```python
from build123d import *

# Parameters (mm, degrees)
SKETCH1_R            = 62.5
BOSS_EXTRUDE8_DEPTH  = 35
BOSS_EXTRUDE9_REACH  = 192.245
SKETCH2_W            = 15
SKETCH2_H            = 35
FILLET4_R            = 10
FILLET5_R            = 10
SKETCH10_W           = 35
SKETCH10_H           = 15
BOSS_EXTRUDE12_DEPTH = 40
SKETCH6_W            = 35
SKETCH6_H            = 15
BOSS_EXTRUDE10_DEPTH = 40
SKETCH12_W           = 42.229373335
SKETCH12_H           = 20
SKETCH12_W_2         = 40
SKETCH12_H_2         = 15
SKETCH12_W_3         = 39.995847529
BOSS_EXTRUDE13_DEPTH = 97.5
SKETCH13_W           = 20
SKETCH13_H           = 5
SKETCH13_W_2         = 25.5
SKETCH13_H_2         = 5.5
BOSS_EXTRUDE14_DEPTH = 20


with BuildPart() as part:
    # Sketch1 → Boss-Extrude8 (new body)
    with BuildSketch(Plane.XY):
        with BuildLine():
            Line((127.600917431, -117.745016448), (72.5, 0))
            ThreePointArc((72.5, 0), (0, 72.5), (-72.5, 0))
            Line((-72.5, 0), (-127.600917431, -117.745016448))
            Line((-127.600917431, -117.745016448), (-167.600917431, -117.745016448))
            Line((-167.600917431, -117.745016448), (-167.600917431, -137.745016448))
            Line((-167.600917431, -137.745016448), (167.600917431, -137.745016448))
            Line((167.600917431, -137.745016448), (167.600917431, -117.745016448))
            Line((167.600917431, -117.745016448), (127.600917431, -117.745016448))
        make_face()
        with BuildLine():
            ThreePointArc((-67.21559633, -27.171926873), (0, -72.5), (67.21559633, -27.171926873))
            Line((67.21559633, -27.171926873), (101.417450928, -100.25778678))
            Line((101.417450928, -100.25778678), (88.408256881, -117.745016448))
            Line((88.408256881, -117.745016448), (-88.408256881, -117.745016448))
            Line((-88.408256881, -117.745016448), (-101.417450928, -100.25778678))
            Line((-101.417450928, -100.25778678), (-67.21559633, -27.171926873))
        make_face(mode=Mode.SUBTRACT)
        Circle(SKETCH1_R, mode=Mode.SUBTRACT)
    extrude(amount=BOSS_EXTRUDE8_DEPTH)

    # Sketch2 → Boss-Extrude9 (add, up to next)
    with BuildSketch(Plane(origin=(0, -117.745016448, 0), x_dir=(1, 0, 0), z_dir=(0, 1, 0)), mode=Mode.PRIVATE) as boss_extrude9_sk1:
        with Locations((0.093911399, -17.5)):
            Rectangle(SKETCH2_W, SKETCH2_H)
    boss_extrude9_tool1 = extrude(boss_extrude9_sk1.sketch, amount=BOSS_EXTRUDE9_REACH, mode=Mode.PRIVATE) - part.part
    add(boss_extrude9_tool1.solids().sort_by_distance((0.093911, -117.745016, 17.5))[0])

    # Fillet4
    fillet4_edges = [part.edges().sort_by_distance(p)[0] for p in [
        (-167.600917431, -117.745016448, 17.5),
    ]]
    fillet(fillet4_edges, radius=FILLET4_R)

    # Fillet5
    fillet5_edges = [part.edges().sort_by_distance(p)[0] for p in [
        (-127.600917431, -117.745016448, 17.5),
    ]]
    fillet(fillet5_edges, radius=FILLET5_R)

    # Sketch10 → Boss-Extrude12 (add)
    with BuildSketch(Plane(origin=(-72.5, 0, 0), x_dir=(0, 0, -1), z_dir=(1, 0, 0))):
        with Locations((-17.5, -7.5)):
            Rectangle(SKETCH10_W, SKETCH10_H)
    extrude(amount=-BOSS_EXTRUDE12_DEPTH)

    # Sketch6 → Boss-Extrude10 (add)
    with BuildSketch(Plane(origin=(72.5, 0, 0), x_dir=(0, 0, -1), z_dir=(1, 0, 0))):
        with Locations((-17.5, -7.5)):
            Rectangle(SKETCH6_W, SKETCH6_H)
    extrude(amount=BOSS_EXTRUDE10_DEPTH)

    # Sketch12 → Boss-Extrude13 (add)
    with BuildSketch(Plane(origin=(0, 0, 0), x_dir=(-1, 0, 0), z_dir=(0, 0, -1))):
        with Locations((-146.486230764, -127.745016448)):
            Rectangle(SKETCH12_W, SKETCH12_H)
        with Locations((147.600917431, -127.745016448)):
            Rectangle(SKETCH12_W_2, SKETCH12_H)
        with Locations((-92.5, -7.5)):
            Rectangle(SKETCH12_W_2, SKETCH12_H_2)
        with Locations((92.502076235, -7.5)):
            Rectangle(SKETCH12_W_3, SKETCH12_H_2)
    extrude(amount=BOSS_EXTRUDE13_DEPTH)

    # Sketch13 → Boss-Extrude14 (add)
    with BuildSketch(Plane(origin=(0, 0, -97.5), x_dir=(-1, 0, 0), z_dir=(0, 0, -1))):
        with Locations((-92.5, -2.5)):
            Rectangle(SKETCH13_W, SKETCH13_H)
        with Locations((-92.5, -12.5)):
            Rectangle(SKETCH13_W, SKETCH13_H)
        with Locations((92.5, -2.5)):
            Rectangle(SKETCH13_W, SKETCH13_H)
        with Locations((92.5, -12.5)):
            Rectangle(SKETCH13_W, SKETCH13_H)
        with Locations((147.600917431, -120.495016448)):
            Rectangle(SKETCH13_W_2, SKETCH13_H_2)
        with Locations((147.600917431, -134.995016448)):
            Rectangle(SKETCH13_W_2, SKETCH13_H_2)
        with Locations((-147.600917431, -120.495016448)):
            Rectangle(SKETCH13_W_2, SKETCH13_H_2)
        with Locations((-147.600917431, -134.995016448)):
            Rectangle(SKETCH13_W_2, SKETCH13_H_2)
    extrude(amount=BOSS_EXTRUDE14_DEPTH)


solid = part.part
```
CAD build for the part. Positions are in the model's coordinates, mm. A direction names the side the tool comes from. Round coordinates to 2 decimals unless told otherwise and drop trailing zeros. Write each loop counter-clockwise with the first axis right and the second up, starting at its lowest first coordinate (ties: lowest second). Pieces come first, ordered by that corner, then holes. Notation, with made-up numbers: (49, 17) - (97, 17) arc R18 ccw to (97, 42) - close; hole circle Ø7 at (-34.75, -39.5). An arc over 180 degrees is marked (long way). Return JSON: item names as keys, results as strings. Group by question number.
Item 1: Mould opens along Y. For faces 5 (the face through (-1, -72, 35)), 6 (the face through (-128.662, -116.225, 17.745)), 7 (the face through (-92, -7, -97.5)) say: +Y half, -Y half, draft (parallel to the pull), parting line (faces both ways), or undercut.
Item 2: Probe probe 1 along Y at (x, z) = (0, 9); probe 2 along Y at (x, z) = (-55, 5.5); probe 3 along X at (y, z) = (-120, -28). List the from-to ranges inside material, lowest first.
Item 3: Band-saw the part on C-C on z = 14.5. List the corners of the cut face in (x, y).
Item 4: Band-saw the part on B-B on z = -7. List the corners of the cut face in (x, y), plus the area to 3 significant figures.
Item 5: 3-axis set-ups, long thin cutter, end or side, ignore diameter. For faces 1 (the face through (-165, -120, 0)), 2 (the face through (148, -123.245, -107)), 3 (the face through (7.594, -95, 18)), 4 (the face through (93, -15, -40)): which of +Z, -Z, +X, -X, +Y, -Y reach the whole face in a straight line?
Item 6: Band-saw the part on A-A on x = 0. List the corners of the cut face in (y, z), plus the area to 3 significant figures.
Item 7: Band-saw the part on D-D on x = -141. List the corners of the cut face in (y, z), plus the area to 3 significant figures.
Item 8: Flat gauge pins, fed straight in: pin 1 Ø16.5 at (y, z) = (-8.5, -59) entering from -X; pin 2 Ø20 at (x, z) = (-140, -34) entering from +Y (3 decimals); pin 3 Ø6 at (x, z) = (-94, -106) entering from +Y. Where does each tip first touch, or does it go through?
Resolved:
{
 "1": {"face 5": "draft", "face 6": "+Y half", "face 7": "undercut"},
 "2": {"probe 1": "y = -137.75 to -62.5, 62.5 to 72.5", "probe 2": "y = -137.75 to -117.75, -47.24 to -29.69, 29.69 to 47.24", "probe 3": "x = -167.6 to -127.6, 125.37 to 167.6"},
 "3": {"outline": "(-167.6, -137.75) - (167.6, -137.75) - (167.6, -117.75) - (127.6, -117.75) - (79.52, -15) - (112.5, -15) - (112.5, 0) - (72.5, 0) arc R72.5 ccw to (-72.5, 0) - (-112.5, 0) - (-112.5, -15) - (-79.52, -15) - (-124.9, -111.98) arc R10 cw to (-133.96, -117.75) - (-157.6, -117.75) arc R10 ccw to (-167.6, -127.75) - close; hole (-101.42, -100.26) - (-88.41, -117.75) - (-7.41, -117.75) - (-7.41, -72.12) arc R72.5 cw to (-67.22, -27.17) - close; hole circle Ø125 at (0, 0); hole (7.59, -117.75) - (88.41, -117.75) - (101.42, -100.26) - (67.22, -27.17) arc R72.5 cw to (7.59, -72.1) - close"},
 "4": {"outline": "(-167.6, -137.75) - (-127.6, -137.75) - (-127.6, -117.75) - (-167.6, -117.75) - close; (-112.5, -15) - (-72.5, -15) - (-72.5, 0) - (-112.5, 0) - close; (72.5, -15) - (112.5, -15) - (112.5, 0) - (72.5, 0) - close; (125.37, -137.75) - (167.6, -137.75) - (167.6, -117.75) - (125.37, -117.75) - close", "area": "2,840 mm²"},
 "5": {"face 1": "+Z, -X, +Y", "face 2": "-Z, +X, -X", "face 3": "+Z, -Z", "face 4": "-Z, +X"},
 "6": {"outline": "(-137.75, 0) - (-62.5, 0) - (-62.5, 35) - (-137.75, 35) - close; (62.5, 0) - (72.5, 0) - (72.5, 35) - (62.5, 35) - close", "area": "2,980 mm²"},
 "7": {"outline": "(-137.75, -117.5) - (-132.25, -117.5) - (-132.25, -97.5) - (-123.25, -97.5) - (-123.25, -117.5) - (-117.75, -117.5) - (-117.75, 35) - (-137.75, 35) - close", "area": "2,870 mm²"},
 "8": {"pin 1": "stops at x = -112.5", "pin 2": "stops at y = -117.745", "pin 3": "stops at y = 0"}
}
